Read the model definition and answer for the solid it produces. Units are mm, in the model's axes. A direction names the side the tool comes from. Coordinates: 2 decimals unless noted, no trailing zeros. Order: outer loops, then holes, each group sorted by start corner. A loop starts at its lowest first (then second) coordinate and runs counter-clockwise, first axis right, second up. Notation, with made-up numbers: M 88,39.5 L 105,39.5 A25 ccw 105,55.5 Z; hole C 59.25,23 d3. An arc over 180 degrees is marked long. Use a Markdown table: item, result. Add a question column.
1) The mould has two halves that part along Y. Classify faces 1 (the face through (8, 0, 22)), 2 (the face through (25, -30, 30)), 3 (the face through (27.2, -22.5, 53.7)): released by +Y, released by -Y, zero draft, split by the parting line, or undercut.
2) Find section A-A on z = 39.5. Write down the section's boundary in (x, y), plus the area to 3 significant figures.
3) Find the intervals of material crossed by probe 1 along Y at (x, z) = (28.5, 66.5); probe 2 along X at (y, z) = (-7.5, 16.5); probe 3 along X at (y, z) = (0, 25.75), in increasing order. Write a range as [from, to].
4) Each of these flat-tipped pins is pushed along its axis until it touches: pin 1 Ø6.5 at (y, z) = (10, 4.5) entering from -X; pin 2 Ø6 at (x, y) = (44.5, 23.5) entering from +Z; pin 3 Ø20 at (x, y) = (48.5, 4) entering from -Z. Where does it stop, or does it pass through?
5) For faces 4 (the face through (44, 0, 12)), 5 (the face through (4, 0, 6)), 6 (the face through (49, 0, 4)), 7 (the face through (27.2, 22.5, 53.7)), 8 (the face through (50, -19, 18)), determine the directions among +Z, -Z, +X, -X, +Y, -Y from which every point of the face is accessible in a straight line to the end or side of a thin tool.
6) Find section D-D on x = 15.5. Write down the section's boundary in (y, z), plus the area to 3 significant figures.
7) Find section B-B on x = 71.5. Write down the section's boundary in (y, z).
8) Find section C-C on y = 5.5. Write down the section's boundary in (x, z).
from build123d import *

# Parameters (mm, degrees)
SKETCH_R        = 9
PAD_DEPTH       = 30
SKETCH001_W     = 55.131706
SKETCH001_H     = 45
POCKET_DEPTH    = 40.001
SKETCH002_R     = 5
POCKET001_DEPTH = 60.001
SKETCH003_R     = 9
POCKET002_DEPTH = 33.001
PAD001_DEPTH    = 12
SKETCH005_W     = 9.754251
SKETCH005_H     = 40
POCKET003_DEPTH = 100.001
SKETCH006_R     = 13
POCKET004_DEPTH = 12
SKETCH007_R     = 8
POCKET005_DEPTH = 12.001


with BuildPart() as part:
    # Sketch → Pad (new body, symmetric)
    with BuildSketch(Plane.XZ):
        with BuildLine():
            Line((0, 0), (70, 0))
            Line((70, 0), (70, 12))
            Line((70, 12), (50, 12))
            Line((50, 12), (50, 25))
            Line((50, 25), (38, 25))
            Line((38, 25), (38, 55))
            ThreePointArc((38, 55), (8, 72.320508), (8, 37.679492))
            Line((8, 6), (8, 37.679492))
            Line((0, 6), (8, 6))
            Line((0, 0), (0, 6))
        make_face()
        with Locations((18, 55)):
            Circle(SKETCH_R, mode=Mode.SUBTRACT)
    extrude(amount=PAD_DEPTH, both=True)

    # Sketch001 → Pocket (cut, through all)
    with BuildSketch(Plane(origin=(38, 0, 0), x_dir=(0, 0, 1), z_dir=(1, 0, 0))):
        with Locations((60.565853, 0)):
            Rectangle(SKETCH001_W, SKETCH001_H)
    extrude(amount=-POCKET_DEPTH, mode=Mode.SUBTRACT)

    # Sketch002 → Pocket001 (cut, through all)
    with BuildSketch(Plane.XZ.offset(30)):
        with Locations((23, 12)):
            Circle(SKETCH002_R)
    extrude(amount=-POCKET001_DEPTH, mode=Mode.SUBTRACT)

    # Sketch003 → Pocket002 (cut, through all)
    with BuildSketch(Plane(origin=(0, 0, 33), x_dir=(-1, 0, 0), z_dir=(0, 0, 1))):
        with Locations((-23, 0)):
            Circle(SKETCH003_R)
    extrude(amount=-POCKET002_DEPTH, mode=Mode.SUBTRACT)

    # Sketch004 → Pad001 (new body)
    with BuildSketch(Plane(origin=(0, 0, 12), x_dir=(-1, 0, 0), z_dir=(0, 0, 1))):
        with BuildLine():
            ThreePointArc((-70, 30), (-100, 0), (-70, -30))
            Line((-70, 30), (-70, -30))
        make_face()
    extrude(amount=-PAD001_DEPTH)

    # Sketch005 → Pocket003 (cut, through all)
    with BuildSketch(Plane(origin=(0, 0, 0), x_dir=(0, 0, -1), z_dir=(-1, 0, 0))):
        with Locations((0.877126, 0)):
            Rectangle(SKETCH005_W, SKETCH005_H)
    extrude(amount=-POCKET003_DEPTH, mode=Mode.SUBTRACT)

    # Sketch006 → Pocket004 (cut)
    with BuildSketch(Plane(origin=(50, 0, 0), x_dir=(0, 0, 1), z_dir=(1, 0, 0))):
        with Locations((25, 0)):
            Circle(SKETCH006_R)
    extrude(amount=-POCKET004_DEPTH, mode=Mode.SUBTRACT)

    # Sketch007 → Pocket005 (cut, through all)
    with BuildSketch(Plane(origin=(0, 0, 12), x_dir=(-1, 0, 0), z_dir=(0, 0, 1))):
        with Locations((-70, 0)):
            Circle(SKETCH007_R)
    extrude(amount=-POCKET005_DEPTH, mode=Mode.SUBTRACT)


solid = part.part
Check result:
| question | item | result |
|---|---|---|
| 1 | face 1 | zero draft |
| 1 | face 2 | released by -Y |
| 1 | face 3 | undercut |
| 2 | outline | M 5.36,-30 L 38,-30 L 38,-22.5 L 5.36,-22.5 Z; M 5.36,22.5 L 38,22.5 L 38,30 L 5.36,30 Z |
| 2 | area | 490 mm2 |
| 3 | probe 1 | y = [-30, -22.5], [22.5, 30] |
| 3 | probe 2 | x = [8, 18.03], [27.97, 38] |
| 3 | probe 3 | x = [8, 14], [32, 38] |
| 4 | pin 1 | stops at x = 0 |
| 4 | pin 2 | stops at z = 25 |
| 4 | pin 3 | stops at z = 4 |
| 5 | face 4 | +Z, +X |
| 5 | face 5 | -X, +Y, -Y |
| 5 | face 6 | -Z, +X, -X |
| 5 | face 7 | +Z, +X, -X |
| 5 | face 8 | +Z, +X, +Y, -Y |
| 6 | outline | M -30,0 L -20,0 L -20,4 L -4.97,4 L -4.97,33 L -22.5,33 L -22.5,46.35 L -30,46.35 Z; M -30,63.65 L -22.5,63.65 L -22.5,74.84 L -30,74.84 Z; M 4.97,4 L 20,4 L 20,0 L 30,0 L 30,46.35 L 22.5,46.35 L 22.5,33 L 4.97,33 Z; M 22.5,63.65 L 30,63.65 L 30,74.84 L 22.5,74.84 Z |
| 6 | area | 1,900 mm2 |
| 7 | outline | M -29.96,0 L -20,0 L -20,4 L -7.86,4 L -7.86,12 L -29.96,12 Z; M 7.86,4 L 20,4 L 20,0 L 29.96,0 L 29.96,12 L 7.86,12 Z |
| 8 | outline | M 0,4 L 15.88,4 L 15.88,33 L 8,33 L 8,6 L 0,6 Z; M 30.12,4 L 64.19,4 L 64.19,12 L 50,12 L 50,13.22 L 38,13.22 L 38,33 L 30.12,33 Z; M 75.81,4 L 99.49,4 L 99.49,12 L 75.81,12 Z |
